Work out the finished part from the listing and answer in its coordinate system (mm). A direction names the side the tool comes from. Round coordinates to 2 decimals unless told otherwise and drop trailing zeros. Write each loop counter-clockwise with the first axis right and the second up, starting at its lowest first coordinate (ties: lowest second). Pieces come first, ordered by that corner, then holes.
1. Find section C-C (x = 0.5). Count the separate pieces of the cut face and the enclosed holes in it, and give its area (3 significant figures).
2. Straight lines are drawn through the part: probe 1 along X at (y, z) = (19, 0); probe 2 along Z at (x, y) = (5.5, 4.5); probe 3 along X at (y, z) = (19.5, 6.75). For each, find the intervals that lie inside material, in ascending order.
3. A tool of negligible diameter and unlimited length cuts with its end or side. For faces 4 (the face through (6, 13, 0)), 5 (the face through (4.132, 20.297, -7.157)), 6 (the face through (-4, 6, -7)), 7 (the face through (-4.31, 16.78, 6.93)), from which of +Z, -Z, +X, -X, +Y, -Y can it reach the whole face along a straight path? Write none if from no direction.
4. Determine the mould class of faces 1 (the face through (5.46, 15.37, -5.22)), 2 (the face through (0.949, 20.297, -10.133)), 3 (the face through (-6.4, 17.97, 8.14)) for opening direction Z: pulls with the +Z half, pulls with the -Z half, needs draft (parallel to the pull), parting line crosses it, or undercut.
5. Flat-ended cylindrical pins translate along their axes: pin 1 Ø12 at (x, y) = (-5, 7.5) entering from +Z; pin 2 Ø6.5 at (y, z) = (7, 1) entering from +X; pin 3 Ø2 at (x, y) = (7.5, 21.5) entering from -Z; pin 4 Ø10 at (x, y) = (6.5, 6.5) entering from +Z. Find the tip coordinate at first contact, or state that the pin passes through.
6. Find section A-A (y = 31). Write down the section's boundary in (x, z) (3 decimals), and give its area (3 significant figures).
7. Find section B-B (z = 3). Write down the section's boundary in (x, y), and give its area (3 significant figures).
```python
from build123d import *

# Parameters (mm, degrees)
RESSALTO_EXTRUS_O1_DEPTH      = 25
ESBO_O3_R                     = 2.25
RESSALTO_EXTRUS_O2_DEPTH      = 3
ESBO_O6_R                     = 1.25
CORTE_EXTRUS_O2_DEPTH         = 10
RESSALTO_EXTRUS_O3_DEPTH      = 5
RESSALTO_EXTRUS_O3_DEPTH_BACK = 7
ESBO_O8_W                     = 16.743157806
ESBO_O8_H                     = 6
CORTE_EXTRUS_O1_DEPTH         = 32.980788504
FILETE2_R                     = 3
ESBO_O10_R                    = 1.75
CORTE_EXTRUS_O3_DEPTH         = 36.379050234
RESSALTO_EXTRUS_O4_DEPTH      = 29
ESBO_O12_R                    = 1.25
CORTE_EXTRUS_O4_DEPTH         = 41.103846452


with BuildPart() as part:
    # Esboço1 → Ressalto-extrusão1 (new body)
    with BuildSketch(Plane(origin=(0, 0, 0), x_dir=(1, 0, 0), z_dir=(0, 1, 0))):
        Polygon((7.25, 4.185789452), (0, 8.371578903), (-7.25, 4.185789452), (-7.25, -4.185789452), (0, -8.371578903), (7.25, -4.185789452), align=None)
    extrude(amount=RESSALTO_EXTRUS_O1_DEPTH)

    # Esboço3 → Ressalto-extrusão2 (add)
    with BuildSketch(Plane(origin=(-3.625, 0, 6.278684177), x_dir=(0.8660254037844387, 0, 0.4999999999999999), z_dir=(-0.49999999999999994, 0, 0.8660254037844388))):
        with Locations(Location((0, 7, 0), (0, 0, 180))):
            Circle(ESBO_O3_R)
        with Locations(Location((0, 18, 0), (0, 0, 180))):
            Circle(ESBO_O3_R)
    extrude(amount=RESSALTO_EXTRUS_O2_DEPTH)

    # Esboço4 → Revolução1 (revolve)
    with BuildSketch(Plane(origin=(0, 18, 0), x_dir=(1, 0, 0), z_dir=(0, 1, 0))):
        Polygon((-7.073557159, -7.751760389), (-6.872595264, -4.403684177), (-5.573557159, -5.153684177), align=None)
    revolve(axis=Axis((-2.565266445, 18, 4.443171818), (-0.5000000000000001, 0, 0.8660254037844386)))

    # Esboço5 → Revolução2 (revolve)
    with BuildSketch(Plane(origin=(0, 7, 0), x_dir=(-1, 0, 0), z_dir=(0, -1, 0)), mode=Mode.PRIVATE) as revolu_o2_sk:
        Polygon((7.073557159, -7.751760389), (5.573557159, -5.153684177), (6.872595264, -4.403684177), align=None)
    revolve(revolu_o2_sk.sketch.rotate(Axis((-5.573557159, 7, 9.653684177), (0.4999999999999998, 0, -0.8660254037844388)), 180), axis=Axis((-5.573557159, 7, 9.653684177), (0.4999999999999998, 0, -0.8660254037844388)))

    # Esboço6 → Corte-extrusão2 (cut)
    with BuildSketch(Plane(origin=(-5.125, 0, 8.876760389), x_dir=(0.8660254037844386, 0, 0.5), z_dir=(-0.5000000000000001, 0, 0.8660254037844387))):
        with Locations((0, 18)):
            Circle(ESBO_O6_R)
        with Locations(Location((0, 7, 0), (0, 0, 180))):
            Circle(ESBO_O6_R)
    extrude(amount=-CORTE_EXTRUS_O2_DEPTH, mode=Mode.SUBTRACT)

    # Esboço8 → Ressalto-extrusão3 (add, two sides: drawn at the far end of the back side and taken through both)
    with BuildSketch(Plane(origin=(3.625, 0, -6.278684177), x_dir=(-0.8660254037844386, 0, -0.4999999999999999), z_dir=(0.49999999999999994, 0, -0.8660254037844387)).offset(-RESSALTO_EXTRUS_O3_DEPTH_BACK)):
        with Locations((0, 3)):
            Rectangle(ESBO_O8_W, ESBO_O8_H)
    extrude(amount=RESSALTO_EXTRUS_O3_DEPTH + RESSALTO_EXTRUS_O3_DEPTH_BACK)

    # Esboço2 → Corte-extrusão1 (cut, through all)
    with BuildSketch(Plane(origin=(0, 25, 0), x_dir=(1, 0, 0), z_dir=(0, 1, 0))):
        Polygon((0, 6.92820323), (-6, 3.464101615), (-6, -3.464101615), (0, -6.92820323), (6, -3.464101615), (6, 3.464101615), align=None)
    extrude(amount=-CORTE_EXTRUS_O1_DEPTH, mode=Mode.SUBTRACT)

    # Filete2
    filete2_edges = [part.edges().sort_by_distance(p)[0] for p in [
        (6.125, 0, -10.608811196),
        (6.125, 6, -10.608811196),
    ]]
    fillet(filete2_edges, radius=FILETE2_R - 0.0001)  # a hair under: the kernel refuses the full size

    # Esboço10 → Corte-extrusão3 (cut, through all)
    with BuildSketch(Plane(origin=(-7.25, 0, -4.185789452), x_dir=(-0.5000000000000001, 0, 0.8660254037844386), z_dir=(-0.8660254037844386, 0, -0.5000000000000001))):
        with Locations((-9.25, 3)):
            Circle(ESBO_O10_R)
    extrude(amount=-CORTE_EXTRUS_O3_DEPTH, mode=Mode.SUBTRACT)

    # Esboço11 → Ressalto-extrusão4 (add)
    with BuildSketch(Plane(origin=(0, 6, 0), x_dir=(1, 0, 0), z_dir=(0, 1, 0))):
        Polygon((-2.625, 12.196524437), (4.625, 8.010734985), (3.625, 6.278684177), (-3.625, 10.464473629), align=None)
    extrude(amount=RESSALTO_EXTRUS_O4_DEPTH)

    # Esboço12 → Corte-extrusão4 (cut, through all)
    with BuildSketch(Plane(origin=(3.625, 0, -6.278684177), x_dir=(0.8660254037844386, 0, 0.4999999999999999), z_dir=(-0.49999999999999994, 0, 0.8660254037844387))):
        with Locations((-4.185789452, 31.5)):
            Circle(ESBO_O12_R)
    extrude(amount=-CORTE_EXTRUS_O4_DEPTH, mode=Mode.SUBTRACT)


solid = part.part
```
Worked answers:
1. separate pieces: 3
1. enclosed holes: 1
1. area: 153 mm2
2. probe 1: x = -7.25 to -6, 6 to 7.25
2. probe 2: z = -10.51 to -8.55, -6.46 to -3.75, 3.75 to 5.2
2. probe 3: x = -6.62 to -0.31, 0.31 to 2.81
3. face 4: +Y, -Y
3. face 5: +X, +Y
3. face 6: -X, +Y
3. face 7: none
4. face 1: undercut
4. face 2: pulls with the -Z half
4. face 3: pulls with the +Z half
5. pin 1: stops at z = 10
5. pin 2: stops at x = 10.87
5. pin 3: stops at z = -4.62
5. pin 4: stops at z = 7.51
6. outline: (-3.625, -10.464) - (-2.625, -12.197) - (0.008, -10.676) - (-0.992, -8.944) - close; (0.992, -7.799) - (1.992, -9.531) - (4.625, -8.011) - (3.625, -6.279) - close
6. area: 12.2 mm2
7. outline: (-7.25, 0) - (-6, 0) - (-6, 25) - (-7.25, 25) - close; (6, 0) - (7.93, 0) - (7.93, 6) - (7.25, 6) - (7.25, 25) - (6, 25) - close
7. area: 66.6 mm2
